from build123d import *

# Parameters (mm, degrees)
SKETCH2_R                = 1.5
BOSS_EXTRUDE1_DEPTH      = 1.5
BOSS_EXTRUDE1_DEPTH_BACK = 1.5
SKETCH3_R                = 1
CUT_EXTRUDE1_DEPTH       = 10


with BuildPart() as part:
    # Sketch1 → Revolve1 (revolve)
    with BuildSketch(Plane.XY):
        Polygon((0, 0), (-5.5, 0), (-5.5, 10), (-4.75, 11), (-4.75, 106), (-5.5, 106), (-5.5, 121), (-3.75, 121), (-3.75, 2), (0, 2), align=None)
    revolve(axis=Axis((0, 121, 0), (0, -1, 0)))

    # Sketch2 → Boss-Extrude1 (add, two sides)
    with BuildSketch(Plane.XY) as boss_extrude1_sk:
        with BuildLine():
            Line((-4, 0), (4, 0))
            Line((4, 0), (4, -5))
            ThreePointArc((4, -5), (0, -9), (-4, -5))
            Line((-4, -5), (-4, 0))
        make_face()
        with Locations((0, -5)):
            Circle(SKETCH2_R, mode=Mode.SUBTRACT)
    extrude(amount=BOSS_EXTRUDE1_DEPTH)
    extrude(boss_extrude1_sk.sketch, amount=-BOSS_EXTRUDE1_DEPTH_BACK)

    # Sketch3 → Cut-Extrude1 (cut)
    with BuildSketch(Plane(origin=(0, 0, 0), x_dir=(0, 0, -1), z_dir=(1, 0, 0))):
        with Locations((0, 3.5)):
            Circle(SKETCH3_R)
        with Locations((0, 113)):
            Circle(SKETCH3_R)
    extrude(amount=CUT_EXTRUDE1_DEPTH, mode=Mode.SUBTRACT)


solid = part.part
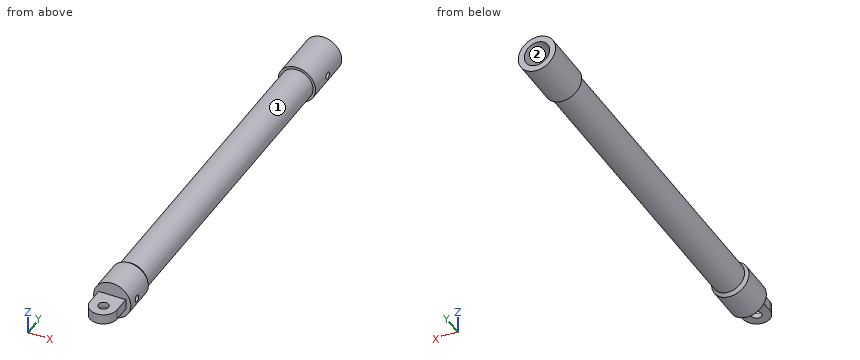
Verification items for the finished model (mm, model axes). Face numbers are marked on the shaded views. Coordinates: 2 decimals unless noted, no trailing zeros. Write each loop counter-clockwise with the first axis right and the second up, starting at its lowest first coordinate (ties: lowest second). Pieces come first, ordered by that corner, then holes. Notation, with made-up numbers: M -2.75,67.5 L 33.25,67.5 A10 ccw 33.25,84.5 Z; hole C 84,-18.75 d5. An arc over 180 degrees is marked long. Use a Markdown table: item, result.
Q1. Thickness scan on line 1 (Y direction, x = 4.7, z = 0); line 2 (Y direction, x = 0, z = -0.5); line 3 (X direction, y = 80, z = 0). Record the ranges inside material, lowest first.
Reply:
| item | result |
|---|---|
| line 1 | y = 0 to 2.5, 4.5 to 112, 114 to 121 |
| line 2 | y = -9 to -6.5, -3.5 to 2 |
| line 3 | x = -4.75 to -3.75, 3.75 to 4.75 |
Q2. Sectioned sample at A-A, the plane x = 0. Record the boundary of the cut face in (y, z), plus the area to 3 significant figures.
Reply:
| item | result |
|---|---|
| outline | M -9,-1.5 L -6.5,-1.5 L -6.5,1.5 L -9,1.5 Z; M -3.5,-1.5 L 0,-1.5 L 0,-5.5 L 10,-5.5 L 11,-4.75 L 106,-4.75 L 106,-5.5 L 121,-5.5 L 121,-3.75 L 2,-3.75 L 2,3.75 L 121,3.75 L 121,5.5 L 106,5.5 L 106,4.75 L 11,4.75 L 10,5.5 L 0,5.5 L 0,1.5 L -3.5,1.5 Z |
| area | 313 mm² |
Q3. Go/stop test with flat-tipped pins: P1, Ø1.5, axis at y = 61.5, z = 0, coming from the +X side; P2, Ø4, axis at x = 0, y = -3.5, coming from the +Z side; P3, Ø3.5, axis at x = -2, z = -2, coming from the -Y side. Record where each tip stops, or that it passes through.
Reply:
| item | result |
|---|---|
| P1 | stops at x = 4.75 |
| P2 | stops at z = 1.5 |
| P3 | stops at y = -8.99 |
Q4. Draft check along Z on the marked faces 1 and 2. Enter one of: +Z half, -Z half, draft (parallel to the pull), parting line (faces both ways), or undercut.
Reply:
| item | result |
|---|---|
| face 1 | parting line |
| face 2 | undercut |
Q5. Sectioned sample at B-B, the plane y = 28. Record the boundary of the cut face in (x, z).
Reply:
| item | result |
|---|---|
| outline | C 0,0 d9.5; hole C 0,0 d7.5 |
